Input: part model. Units: mm. Frame: model coordinates. A direction names the side the tool comes from. Round coordinates to 2 decimals unless told otherwise and drop trailing zeros. Order: outer loops, then holes, each group sorted by start corner. A loop starts at its lowest first (then second) coordinate and runs counter-clockwise, first axis right, second up. Notation, with made-up numbers: (27.25, 49) -> (72.25, 49) arc R28 ccw to (72.25, 68) -> close; hole circle Ø10 at (48, 63). An arc over 180 degrees is marked (long way). Answer as CSV lines item,"result". Start each with the question number.
1) First-contact query: P1, Ø0.6, axis at x = -4, z = 15, coming from the +Y side; P2, Ø1.6, axis at x = -15.5, z = 7, coming from the +Y side. Flat tips, straight axial feed; report the tip coordinate or a pass-through.
2) Access query for faces 4 (the face through (-10, -8.381, 11)), 5 (the face through (-2.89, -6.167, 6.513)), 6 (the face through (-6.066, -9.3, 11.1)). Directions: +Z, -Z, +X, -X, +Y, -Y. A direction counts if a zero-diameter tool reaches every point of the face in a straight line with its end or side. Return the directions, or none.
3) Section query D-D, the plane x = -9.25. Output: boundary loops of the cut face in (y, z).
4) Section query A-A, the plane y = -9.2. Output: boundary loops of the cut face in (x, z), and give its area (3 significant figures).
5) Mould query, pull axis Y, two halves, no side actions, for faces 1 (the face through (-6.6, -9.681, 11.1)), 2 (the face through (-18.066, -8, 11)), 3 (the face through (-15, -10.481, 11)). Classes: +Y half, -Y half, draft (parallel to the pull), parting line (faces both ways), or undercut.
6) Line query: L1, parallel to X at y = -6.15, z = 15.25; L2, parallel to Y at x = -6.25, z = 1.5; L3, parallel to X at y = -8.75, z = 12. Output: solid intervals per line, ascending.
7) Section query B-B, the plane z = 12.5. Output: boundary loops of the cut face in (x, y), and give its area (3 significant figures).
8) Section query C-C, the plane y = -6.7. Output: boundary loops of the cut face in (x, z), and give its area (3 significant figures).
```python
from build123d import *

# Parameters (mm, degrees)
EXTRUDE_1_DEPTH     = 22.5
SKETCH_4_R          = 1
CUT_EXTRUDE_4_DEPTH = 2


with BuildPart() as part:
    # 草图1 → 凸台-拉伸1 (new body)
    with BuildSketch(Plane.XY):
        Polygon((-18.065809082, -5.18088445), (-18.065809082, -10.48088445), (-12.065809082, -10.48088445), (-12.065809082, -9.68088445), (-13.065809082, -9.68088445), (-13.065809082, -8.88088445), (-12.065809082, -8.88088445), (-12.065809082, -8.38088445), (-9.565809082, -8.38088445), (-9.565809082, -5.18088445), align=None)
        Polygon((-1.065809082, -5.18088445), (-9.565809082, -5.18088445), (-9.565809082, -8.38088445), (-7.065809082, -8.38088445), (-7.065809082, -8.88088445), (-6.065809082, -8.88088445), (-6.065809082, -9.68088445), (-7.065809082, -9.68088445), (-7.065809082, -10.48088445), (-1.065809082, -10.48088445), align=None)
    extrude(amount=EXTRUDE_1_DEPTH)

    # 草图4 → 切除-拉伸4 (cut)
    with BuildSketch(Plane(origin=(0, -5.18088445, 0), x_dir=(1, 0, 0), z_dir=(0, 1, 0))):
        with Locations(Location((-15.565809082, -7.25, 0), (0, 0, 270))):
            Circle(SKETCH_4_R)
        with Locations(Location((-15.565809082, -15.25, 0), (0, 0, 270))):
            Circle(SKETCH_4_R)
        with Locations(Location((-3.565809082, -7.25, 0), (0, 0, 270))):
            Circle(SKETCH_4_R)
        with Locations(Location((-3.565809082, -15.25, 0), (0, 0, 270))):
            Circle(SKETCH_4_R)
    extrude(amount=-CUT_EXTRUDE_4_DEPTH, mode=Mode.SUBTRACT)


solid = part.part
```
Findings:
1,P1,"stops at y = -7.18"
1,P2,"stops at y = -5.18"
2,face 4,"+Z, -Z, -Y"
2,face 5,"+Y"
2,face 6,"+Z, -Z"
3,outline,"(-8.38, 0) -> (-5.18, 0) -> (-5.18, 22.5) -> (-8.38, 22.5) -> close"
4,outline,"(-18.07, 0) -> (-13.07, 0) -> (-13.07, 22.5) -> (-18.07, 22.5) -> close; (-6.07, 0) -> (-1.07, 0) -> (-1.07, 22.5) -> (-6.07, 22.5) -> close"
4,area,"225 mm^2"
5,face 1,"undercut"
5,face 2,"draft"
5,face 3,"-Y half"
6,L1,"x = -18.07 to -16.57, -14.57 to -4.57, -2.57 to -1.07"
6,L2,"y = -10.48 to -9.68, -8.88 to -5.18"
6,L3,"x = -18.07 to -12.07, -7.07 to -1.07"
7,outline,"(-18.07, -10.48) -> (-12.07, -10.48) -> (-12.07, -9.68) -> (-13.07, -9.68) -> (-13.07, -8.88) -> (-12.07, -8.88) -> (-12.07, -8.38) -> (-7.07, -8.38) -> (-7.07, -8.88) -> (-6.07, -8.88) -> (-6.07, -9.68) -> (-7.07, -9.68) -> (-7.07, -10.48) -> (-1.07, -10.48) -> (-1.07, -5.18) -> (-18.07, -5.18) -> close"
7,area,"78.0 mm^2"
8,outline,"(-18.07, 0) -> (-1.07, 0) -> (-1.07, 22.5) -> (-18.07, 22.5) -> close; hole circle Ø2 at (-15.57, 7.25); hole circle Ø2 at (-15.57, 15.25); hole circle Ø2 at (-3.57, 7.25); hole circle Ø2 at (-3.57, 15.25)"
8,area,"370 mm^2"
